from build123d import *

# Parameters (mm, degrees)
CORTAR_EXTRUIR1_DEPTH      = 36.010034276
CORTAR_EXTRUIR1_DEPTH_BACK = 36.010034276
CROQUIS2_W                 = 30
CROQUIS2_H                 = 1


with BuildPart() as part:
    # Croquis1 → Revolución1 (revolve)
    with BuildSketch(Plane(origin=(0, 0, 0), x_dir=(1, 0, 0), z_dir=(0, 1, 0)), mode=Mode.PRIVATE) as revoluci_n1_sk:
        Polygon((-34.55, 0), (-34.55, 4), (-31.55, 4), (-31.55, 3), (-30.55, 3), (-30.55, 4), (30.55, 4), (30.55, 3), (31.55, 3), (31.55, 4), (34.55, 4), (34.55, 0), align=None)
    revolve(revoluci_n1_sk.sketch.rotate(Axis((-34.55, 0, 0), (1, 0, 0)), 180), axis=Axis((-34.55, 0, 0), (1, 0, 0)))

    # Croquis2 → Cortar-Extruir1 (cut, two sides: drawn at the far end of the back side and taken through both)
    with BuildSketch(Plane(origin=(0, 0, 0), x_dir=(1, 0, 0), z_dir=(0, 1, 0)).offset(-CORTAR_EXTRUIR1_DEPTH_BACK)):
        with Locations((-15.55, -3.5)):
            Rectangle(CROQUIS2_W, CROQUIS2_H)
    extrude(amount=CORTAR_EXTRUIR1_DEPTH + CORTAR_EXTRUIR1_DEPTH_BACK, mode=Mode.SUBTRACT)


solid = part.part
Verification items for the finished model (mm, model axes). A direction names the side the tool comes from. Coordinates: 2 decimals unless noted, no trailing zeros. Write each loop counter-clockwise with the first axis right and the second up, starting at its lowest first coordinate (ties: lowest second). Pieces come first, ordered by that corner, then holes. Notation, with made-up numbers: (-23, 52.5) -> (-11, 52.5) arc R25 ccw to (-11, 73.5) -> close; hole circle Ø8 at (75.5, -8). An arc over 180 degrees is marked (long way). One line per item, written item: value. Start each with the question number.
Q1. Cross-section at A-A on y = 2. Enter the section's corners in (x, z), and give its area (3 significant figures).
Q2. Cross-section at D-D on x = -17. Enter the section's corners in (y, z).
Q3. Go/stop test with flat-tipped pins: P1, Ø1, axis at x = 24, y = -1.5, coming from the +Z side; P2, Ø2.5, axis at x = -11.5, y = -0.5, coming from the +Z side; P3, Ø1, axis at x = 14.5, y = 2.5, coming from the -Z side. Record where each tip stops, or that it passes through.
Q4. Mould release check, pull along X, two halves, no side actions. Record for faces 1 (the flat face through (-31.55, -3, 1)), 2 (the flat face through (-34.55, 0, 0)), 3 (the flat face through (34.55, 0, 0)): pulls with the +X half, pulls with the -X half, needs draft (parallel to the pull), parting line crosses it, or undercut.
Q5. Cross-section at C-C on z = -1.75. Enter the section's corners in (x, y), and give its area (3 significant figures).
Q6. Access from +Z, -Z, +X, -X, +Y, -Y to the whole of each face (thin tool, end or side, straight path). Record for faces 4 (the cylindrical face through (33.071, 3.905, -0.867)), 5 (the flat face through (-16, 0, 3)), 6 (the cylindrical face through (31.06, -0.9, 2.86)).
Q7. Thickness scan on L1, parallel to X at y = 3, z = 1.75; L2, parallel to Y at x = -21.5, z = 0.25; L3, parallel to Z at x = -14, y = -0.25. Record the ranges inside material, lowest first. Write a range as from..to.
Q8. Cross-section at B-B on x = 1. Enter the section's corners in (y, z).
Checked values:
1. outline: (-34.55, -3.46) -> (-31.55, -3.46) -> (-31.55, -2.24) -> (-30.55, -2.24) -> (-30.55, -3.46) -> (30.55, -3.46) -> (30.55, -2.24) -> (31.55, -2.24) -> (31.55, -3.46) -> (34.55, -3.46) -> (34.55, 3.46) -> (31.55, 3.46) -> (31.55, 2.24) -> (30.55, 2.24) -> (30.55, 3.46) -> (-0.55, 3.46) -> (-0.55, 3) -> (-30.55, 3) -> (-30.55, 2.24) -> (-31.55, 2.24) -> (-31.55, 3.46) -> (-34.55, 3.46) -> close
1. area: 460 mm²
2. outline: (-2.65, 3) arc R4 ccw (long way) to (2.65, 3) -> close
3. P1: stops at z = 3.87
3. P2: stops at z = 3
3. P3: stops at z = -3.46
4. face 1: undercut
4. face 2: pulls with the -X half
4. face 3: pulls with the +X half
5. outline: (-34.55, -3.6) -> (-31.55, -3.6) -> (-31.55, -2.44) -> (-30.55, -2.44) -> (-30.55, -3.6) -> (30.55, -3.6) -> (30.55, -2.44) -> (31.55, -2.44) -> (31.55, -3.6) -> (34.55, -3.6) -> (34.55, 3.6) -> (31.55, 3.6) -> (31.55, 2.44) -> (30.55, 2.44) -> (30.55, 3.6) -> (-30.55, 3.6) -> (-30.55, 2.44) -> (-31.55, 2.44) -> (-31.55, 3.6) -> (-34.55, 3.6) -> close
5. area: 492 mm²
6. face 4: +X, -X
6. face 5: +Z, +Y, -Y
6. face 6: none
7. L1: x = -34.55..-31.55, -30.55..30.55, 31.55..34.55
7. L2: y = -3.99..3.99
7. L3: z = -3.99..3
8. outline: circle Ø8 at (0, 0)
